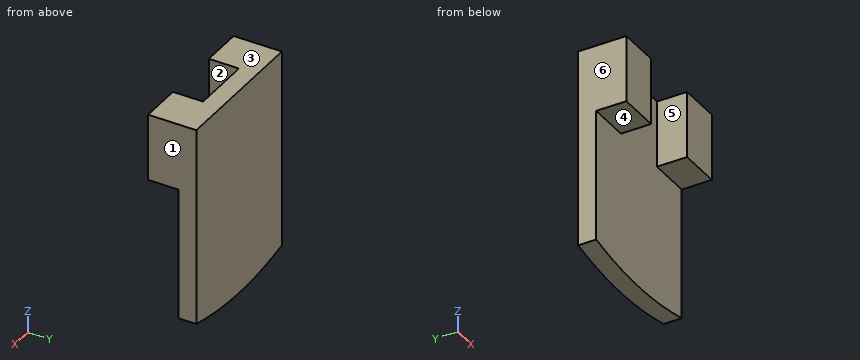
```python
from build123d import *

# Parameters (mm, degrees)
BOSS_EXTRUDE1_DEPTH = 3
SKETCH4_W           = 24
SKETCH4_H           = 0.6
CUT_EXTRUDE3_DEPTH  = 4.0000001
SKETCH5_W           = 6.959988298
SKETCH5_H           = 11.094755151
BOSS_EXTRUDE2_DEPTH = 5


with BuildPart() as part:
    # Sketch1 → Boss-Extrude1 (new body)
    with BuildSketch(Plane(origin=(0, 0, 0), x_dir=(1, 0, 0), z_dir=(0, 1, 0))):
        with BuildLine():
            Line((0, 0), (24, 0))
            Line((24, 0), (24, 33.6))
            add(Edge.make_bspline(
                [(0, 33.6), (12, 36.4), (24, 33.6)],
                knots=[0, 0, 0, 1, 1, 1], degree=2))
            Line((0, 33.6), (0, 0))
        make_face()
    extrude(amount=BOSS_EXTRUDE1_DEPTH)

    # Sketch4 → Cut-Extrude3 (cut, through all)
    with BuildSketch(Plane(origin=(0, 3, 0), x_dir=(1, 0, 0), z_dir=(0, 1, 0))):
        with Locations((12, 0.3)):
            Rectangle(SKETCH4_W, SKETCH4_H)
    extrude(amount=-CUT_EXTRUDE3_DEPTH, mode=Mode.SUBTRACT)

    # Sketch5 → Boss-Extrude2 (add)
    with BuildSketch(Plane.XZ):
        with Locations((3.479994149, -6.147377576)):
            Rectangle(SKETCH5_W, SKETCH5_H)
        with Locations((20.520005851, -6.147377576)):
            Rectangle(SKETCH5_W, SKETCH5_H)
    extrude(amount=BOSS_EXTRUDE2_DEPTH)


solid = part.part
```
Here's how the part is built. I have some questions about the finished solid (model axes, mm). Face numbers are marked on the shaded views. A direction names the side the tool comes from. Round coordinates to 2 decimals unless told otherwise and drop trailing zeros. Loops run counter-clockwise (first coordinate to the right, second up) from the corner with the lowest first, then second, coordinate; pieces in that order, holes last. Notation, with made-up numbers: (7.25, 82) -> (58.25, 82) arc R20 ccw to (58.25, 95) -> close; hole circle Ø9 at (-11.5, 30.25). An arc over 180 degrees is marked (long way). Answer as CSV lines item,"result".
1. If I drill on L1, parallel to X at y = -4.25, z = -5.5; L2, parallel to Y at x = 12, z = -21.5; L3, parallel to Z at x = 2, y = -3.75, over which ranges is the centre line in solid material (lowest first)?
Final values:
L1,"x = 0 to 6.96, 17.04 to 24"
L2,"y = 0 to 3"
L3,"z = -11.69 to -0.6"
2. If we section it at A-A on y = -3.5: Please give me the cut outline in (x, z).
Final values:
outline,"(0, -11.69) -> (6.96, -11.69) -> (6.96, -0.6) -> (0, -0.6) -> close; (17.04, -11.69) -> (24, -11.69) -> (24, -0.6) -> (17.04, -0.6) -> close"
3. Which directions (+Z, -Z, +X, -X, +Y, -Y) give clear straight access to the entire face, cutting with the end or side of a thin tool? Please do the marked faces 4, 5 and 6.
Final values:
face 4,"-Z, +X, -X, -Y"
face 5,"+Z, -Z, -Y"
face 6,"+Z, -Z, -X, +Y, -Y"
4. If we section it at B-B on z = -3: Please give me the cut outline in (x, y), plus the area to 3 significant figures.
Final values:
outline,"(0, -5) -> (6.96, -5) -> (6.96, 0) -> (17.04, 0) -> (17.04, -5) -> (24, -5) -> (24, 3) -> (0, 3) -> close"
area,"142 mm^2"
5. Thinking about a two-plate mould opening in X: for the marked faces 1, 2 and 3, which applies, released by +X, released by -X, zero draft, split by the parting line, or undercut?
Final values:
face 1,"released by +X"
face 2,"undercut"
face 3,"zero draft"
6. For pin 1 (12 mm diameter, centred on x = 20.5, z = -25.5, fed in from -Y); pin 2 (1.5 mm diameter, centred on x = 19, y = -1.5, fed in from -Z); pin 3 (2 mm diameter, centred on x = 9, y = -1.5, fed in from -Z), each with a flat end and sliding along its axis, tell me the tip position at first contact or that it passes through.
Final values:
pin 1,"stops at y = 0"
pin 2,"stops at z = -11.69"
pin 3,"passes through"
7. If we section it at C-C on z = -15.5: Please give me the cut outline in (x, y), plus the area to 3 significant figures.
Final values:
outline,"(0, 0) -> (24, 0) -> (24, 3) -> (0, 3) -> close"
area,"72.0 mm^2"
